Part model, mm, in its own coordinate system. Round coordinates to 2 decimals unless told otherwise and drop trailing zeros. Loops run counter-clockwise (first coordinate to the right, second up) from the corner with the lowest first, then second, coordinate; pieces in that order, holes last. Notation, with made-up numbers: (57, 63.25) -> (68, 63.25) arc R17 ccw to (68, 91.25) -> close; hole circle Ø7 at (39, 18). An arc over 180 degrees is marked (long way). Answer as CSV lines item,"result".
from build123d import *

# Parameters (mm, degrees)
F0_W     = 76.2
F0_H     = 76.2
F0_R     = 19.05
F1_DEPTH = 22.225
F2_R     = 5.08


with BuildPart() as f1:
    # F0 (on Front) → F1 (new body, symmetric)
    with BuildSketch(Plane.XZ):
        Rectangle(F0_W, F0_H)
        Circle(F0_R, mode=Mode.SUBTRACT)
    extrude(amount=F1_DEPTH, both=True)

    # F2
    f2_edges = [f1.edges().sort_by_distance(p)[0] for p in [
        (38.1, 0, 38.1),
        (-38.1, 0, 38.1),
        (38.1, 0, -38.1),
        (-38.1, 0, -38.1),
        (-19.05, -22.225, 0),
        (-19.05, 22.225, 0),
    ]]
    fillet(f2_edges, radius=F2_R)


solid = f1.part
Q1. Saw through at A-A, the plane z = 0. Write the cut outline in (x, y) (3 decimals).
Geometry results:
outline,"(-38.1, -22.225) -> (-24.13, -22.225) arc R5.08 ccw to (-19.05, -17.145) -> (-19.05, 17.145) arc R5.08 ccw to (-24.13, 22.225) -> (-38.1, 22.225) -> close; (19.05, -17.145) arc R5.08 ccw to (24.13, -22.225) -> (38.1, -22.225) -> (38.1, 22.225) -> (24.13, 22.225) arc R5.08 ccw to (19.05, 17.145) -> close"
Q2. Drill centre lines: line 1 along Z through (x, y) = (0, -3); line 2 along X through (y, z) = (3.5, 4); line 3 along X through (y, z) = (12.5, -16). Where is each one in solid material? Low to high.
Geometry results:
line 1,"-38.1 to -19.05, 19.05 to 38.1"
line 2,"-38.1 to -18.63, 18.63 to 38.1"
line 3,"-38.1 to -10.34, 10.34 to 38.1"
Q3. Saw through at C-C, the plane y = -15. Write the cut outline in (x, z), then the cut area to 3 significant figures.
Geometry results:
outline,"(-38.1, -33.02) arc R5.08 ccw to (-33.02, -38.1) -> (33.02, -38.1) arc R5.08 ccw to (38.1, -33.02) -> (38.1, 33.02) arc R5.08 ccw to (33.02, 38.1) -> (-33.02, 38.1) arc R5.08 ccw to (-38.1, 33.02) -> close; hole circle Ø38.1 at (0, 0)"
area,"4,640 mm2"
Q4. Saw through at B-B, the plane x = 0. Write the cut outline in (y, z) (3 decimals), then the cut area to 3 significant figures.
Geometry results:
outline,"(-22.225, -38.1) -> (22.225, -38.1) -> (22.225, -24.13) arc R5.08 ccw to (17.145, -19.05) -> (-17.145, -19.05) arc R5.08 ccw to (-22.225, -24.13) -> close; (-22.225, 24.13) arc R5.08 ccw to (-17.145, 19.05) -> (17.145, 19.05) arc R5.08 ccw to (22.225, 24.13) -> (22.225, 38.1) -> (-22.225, 38.1) -> close"
area,"1,670 mm2"
Q5. Two-plate mould, pull along Z, no slides. Class faces 1 (the face through (-36.651, -0.311, -36.572)), 2 (the face through (38.1, 0, 0)), 3 (the face through (-15.12, 0.24, -11.59)), 4 (the face through (0, 0, 38.1)): pulls with the +Z half, pulls with the -Z half, needs draft (parallel to the pull), parting line crosses it, or undercut.
Geometry results:
face 1,"pulls with the -Z half"
face 2,"needs draft"
face 3,"undercut"
face 4,"pulls with the +Z half"
